Check sheet for the modelled part. Datum: model origin and axes. Units: mm. A direction names the side the tool comes from. Round coordinates to 2 decimals unless told otherwise and drop trailing zeros. Order: outer loops, then holes, each group sorted by start corner. A loop starts at its lowest first (then second) coordinate and runs counter-clockwise, first axis right, second up.
(1) Mould release check, pull along Z, two halves, no side actions. Record for faces 4 (the flat face through (56, 0, 12)), 5 (the cylindrical face through (-15.12, -18.78, -11.59)), 6 (the flat face through (64.525, -12.522, -19.043)): released by +Z, released by -Z, zero draft, split by the parting line, or undercut.
(2) Thickness scan on probe 1 along X at (y, z) = (-27.5, -11); probe 2 along Y at (x, z) = (63, -13.5); probe 3 along Z at (x, y) = (0, -22). Record the ranges inside material, lowest first.
(3) Sectioned sample at A-A, the plane x = 0. Enter the section's corners in (y, z).
(4) Sectioned sample at C-C, the plane y = -17. Enter the section's corners in (x, z).
(5) Tool access check on faces 1 (the flat face through (4, -38.1, 19)), 2 (the flat face through (130, -31.75, 6)), 3 (the cylindrical face through (31.75, -12.52, -0.14)). Record the directions out of +Z, -Z, +X, -X, +Y, -Y that give a thin tool (end or side, any length) a straight path to the whole face; none if there is none.
(6) Sectioned sample at B-B, the plane z = 17.5. Enter the section's corners in (x, y), and give its area (3 significant figures).
(7) Sectioned sample at D-D, the plane x = 63. Enter the section's corners in (y, z), and give its area (3 significant figures).
(8) Depth check by flat-ended pin: pin 1 (5 mm diameter, centred on x = 106, z = -4, fed in from +Y); pin 2 (7.5 mm diameter, centred on x = 65, y = -16.5, fed in from +Z); pin 3 (3 mm diameter, centred on y = -11.5, z = -3.5, fed in from -X); pin 4 (6 mm diameter, centred on y = -27, z = 10.5, fed in from +X). Enter the tip coordinate at first touch or a pass-through.
```python
from build123d import *

# Parameters (mm, degrees)
F0_R     = 19.05
F1_DEPTH = 38.1
F2_DEPTH = 25.4
F0_R_2   = 6.35
F3_DEPTH = 31.75


with BuildPart() as f1:
    # F0 (on Front) → F1 (new body)
    with BuildSketch(Plane.XZ):
        with BuildLine():
            ThreePointArc((2.540001, -25.272681), (18.837144, -17.038838), (25.4, 0))
            ThreePointArc((25.4, 0), (18.841479, 17.034044), (2.552862, 25.271385))
            ThreePointArc((2.552862, 25.271385), (-25.399999, 0.006463), (2.540001, -25.272681))
        make_face()
        Circle(F0_R, mode=Mode.SUBTRACT)
    extrude(amount=F1_DEPTH)

    # F0 (on Front) → F2 (join)
    with BuildSketch(Plane.XZ):
        with BuildLine():
            ThreePointArc((2.552862, 25.271385), (18.841479, 17.034044), (25.4, 0))
            ThreePointArc((25.4, 0), (18.837144, -17.038838), (2.540001, -25.272681))
            Line((2.540001, -25.272681), (128.27, -12.63634))
            ThreePointArc((128.27, -12.63634), (114.315925, -0.635797), (127, 12.7))
            Line((127, 12.7), (2.552862, 25.271385))
        make_face()
        with BuildLine():
            ThreePointArc((38.1, -6.35), (31.75, 0), (38.1, 6.35))
            Line((38.1, 6.35), (88.9, 6.35))
            ThreePointArc((88.9, 6.35), (95.25, 0), (88.9, -6.35))
            Line((88.9, -6.35), (38.1, -6.35))
        make_face(mode=Mode.SUBTRACT)
    extrude(amount=F2_DEPTH)

    # F0 (on Front) → F3 (join)
    with BuildSketch(Plane.XZ):
        with BuildLine():
            ThreePointArc((139.7, 0), (135.980256, 8.980256), (127, 12.7))
            ThreePointArc((127, 12.7), (114.315925, -0.635797), (128.27, -12.63634))
            ThreePointArc((128.27, -12.63634), (136.418572, -8.519419), (139.7, 0))
        make_face()
        with Locations((127, 0)):
            Circle(F0_R_2, mode=Mode.SUBTRACT)
    extrude(amount=F3_DEPTH)


solid = f1.part
```
Derived:
1. face 4: zero draft
1. face 5: undercut
1. face 6: released by -Z
2. probe 1: x = -22.89 to -15.55, 15.55 to 22.89, 120.65 to 133.35
2. probe 2: y = -25.4 to 0
2. probe 3: z = -25.4 to -19.05, 19.05 to 25.4
3. outline: (-38.1, -25.4) - (0, -25.4) - (0, -19.05) - (-38.1, -19.05) - close; (-38.1, 19.05) - (0, 19.05) - (0, 25.4) - (-38.1, 25.4) - close
4. outline: (2.54, -25.27) - (128.27, -12.64) arc R12.7 ccw to (139.7, 0) arc R12.7 ccw to (127, 12.7) - (2.55, 25.27) arc R25.4 ccw (long way) to start; hole circle Ø38.1 at (0, 0); hole (38.1, -6.35) - (88.9, -6.35) arc R6.35 ccw to (88.9, 6.35) - (38.1, 6.35) arc R6.35 ccw to start; hole circle Ø12.7 at (127, 0)
5. face 1: +Z, -Z, +X, -X, -Y
5. face 2: +Z, -Z, +X, -Y
5. face 3: +Y, -Y
6. outline: (-18.41, -38.1) - (-7.53, -38.1) - (-7.53, 0) - (-18.41, 0) - close; (7.53, -38.1) - (18.41, -38.1) - (18.41, -25.4) - (79.48, -25.4) - (79.48, 0) - (7.53, 0) - close
6. area: 2,380 mm2
7. outline: (-25.4, -19.2) - (0, -19.2) - (0, -6.35) - (-25.4, -6.35) - close; (-25.4, 6.35) - (0, 6.35) - (0, 19.17) - (-25.4, 19.17) - close
7. area: 652 mm2
8. pin 1: stops at y = 0
8. pin 2: stops at z = 19.34
8. pin 3: stops at x = -25.32
8. pin 4: stops at x = 137.25
